Work out the finished part from the listing and answer in its coordinate system (mm). A direction names the side the tool comes from. Give positions to 0.01 mm unless a question says otherwise; leave off trailing zeros. Write each loop counter-clockwise with the first axis right and the second up, starting at its lowest first coordinate (ties: lowest second). Pieces come first, ordered by that corner, then holes. Notation, with made-up numbers: (-9, -8) -> (10, -8) arc R21 ccw to (10, 0) -> close; hole circle Ø3 at (83.5, 13.25). An arc over 180 degrees is marked (long way). Use a Markdown table: item, result. Add a question column.
Q1. Consider line 1 (Z direction, x = 0, y = 4.25) (3 decimals); line 2 (Y direction, x = -4.75, z = -1); line 3 (Z direction, x = 2, y = 2.25). Determine where each line is inside the solid, lowest interval first.
Q2. For faces 1 (the face through (-1, 1.626, 4)), 2 (the face through (3, 0, -1)), determine the directions among +Z, -Z, +X, -X, +Y, -Y from which every point of the face is accessible in a straight line to the end or side of a thin tool.
Q3. Section A-A, the plane x = 0 is taken. Give the vertices of the cut face in (y, z) (3 decimals).
Q4. Section B-B, the plane z = 0 is taken. Give the vertices of the cut face in (x, y) (3 decimals), plus the area to 3 significant figures.
Q5. Section C-C, the plane y = 3.25 is taken. Give the vertices of the cut face in (x, z) (3 decimals), plus the area to 3 significant figures.
Q6. Each of these flat-tipped pins is pushed along its axis until it touches: pin 1 Ø1 at (x, y) = (0, 6.5) entering from +Z (3 decimals); pin 2 Ø4 at (x, z) = (0, 0) entering from -Y; pin 3 Ø2 at (x, y) = (-1, 5.5) entering from -Z (3 decimals). Where does it stop, or does it pass through?
Q7. For a pull along Z with two mould halves and no side action, classify faces 3 (the face through (-2.893, 4.933, 2.653)), 4 (the face through (1.29, 4.119, 2.024)), 5 (the face through (2, 8.4, -2)) as pulls with the +Z half, pulls with the -Z half, needs draft (parallel to the pull), parting line crosses it, or undercut.
Q8. Section D-D, the plane x = 4.25 is taken. Give the vertices of the cut face in (y, z), plus the area to 3 significant figures.
from build123d import *

# Parameters (mm, degrees)
SKETCH2_W               = 14
SKETCH2_H               = 8
CUT_EXTRUDE1_DEPTH      = 6.5
CUT_EXTRUDE1_DEPTH_BACK = 6.5
CHAMFER1_SIZE           = 0.25


with BuildPart() as part:
    # Sketch1 → Revolve1 (revolve)
    with BuildSketch(Plane.XY):
        Polygon((3.925, 1.6256), (3.925, 12.4), (2.4, 12.4), (2.4, 0.2), (2.6, 0), (5.5, 0), (5.5, 1.6256), align=None)
    revolve(axis=Axis((0, 0, 0), (0, -1, 0)))

    # Sketch2 → Cut-Extrude1 (cut, two sides)
    with BuildSketch(Plane.XY) as cut_extrude1_sk:
        with Locations((0, 12.4)):
            Rectangle(SKETCH2_W, SKETCH2_H)
    extrude(amount=CUT_EXTRUDE1_DEPTH, mode=Mode.SUBTRACT)
    extrude(cut_extrude1_sk.sketch, amount=-CUT_EXTRUDE1_DEPTH_BACK, mode=Mode.SUBTRACT)

    # Chamfer1
    chamfer1_edges = [part.edges().sort_by_distance(p)[0] for p in [
        (-3.925, 8.4, 0),
        (-2.4, 8.4, 0),
    ]]
    chamfer(chamfer1_edges, length=CHAMFER1_SIZE)


solid = part.part
Result set:
| question | item | result |
|---|---|---|
| 1 | line 1 | z = -3.925 to -2.4, 2.4 to 3.925 |
| 1 | line 2 | y = 0 to 1.63 |
| 1 | line 3 | z = -3.38 to -1.33, 1.33 to 3.38 |
| 2 | face 1 | +Y |
| 2 | face 2 | +Z, -Z, +X, -X, -Y |
| 3 | outline | (0, -5.5) -> (1.626, -5.5) -> (1.626, -3.925) -> (8.15, -3.925) -> (8.4, -3.675) -> (8.4, -2.65) -> (8.15, -2.4) -> (0.2, -2.4) -> (0, -2.6) -> close; (0, 2.6) -> (0.2, 2.4) -> (8.15, 2.4) -> (8.4, 2.65) -> (8.4, 3.675) -> (8.15, 3.925) -> (1.626, 3.925) -> (1.626, 5.5) -> (0, 5.5) -> close |
| 4 | outline | (-5.5, 0) -> (-2.6, 0) -> (-2.4, 0.2) -> (-2.4, 8.15) -> (-2.65, 8.4) -> (-3.675, 8.4) -> (-3.925, 8.15) -> (-3.925, 1.626) -> (-5.5, 1.626) -> close; (2.4, 0.2) -> (2.6, 0) -> (5.5, 0) -> (5.5, 1.626) -> (3.925, 1.626) -> (3.925, 8.15) -> (3.675, 8.4) -> (2.65, 8.4) -> (2.4, 8.15) -> close |
| 4 | area | 30.6 mm2 |
| 5 | outline | circle Ø7.85 at (0, 0); hole circle Ø4.8 at (0, 0) |
| 5 | area | 30.3 mm2 |
| 6 | pin 1 | stops at z = 3.925 |
| 6 | pin 2 | passes through |
| 6 | pin 3 | stops at z = -3.925 |
| 7 | face 3 | parting line crosses it |
| 7 | face 4 | undercut |
| 7 | face 5 | needs draft |
| 8 | outline | (0, -3.49) -> (1.63, -3.49) -> (1.63, 3.49) -> (0, 3.49) -> close |
| 8 | area | 11.4 mm2 |
